Verification items for the finished model (mm, model axes). Coordinates: 2 decimals unless noted, no trailing zeros. Answer in a Markdown table with one row per item.
from build123d import *

# Parameters (mm, degrees)
F0_W     = 1375.41
F0_H     = 16.002
F0_R     = 2.286
F1_DEPTH = 3.175


with BuildPart() as f1:
    # F0 (on Top) → F1 (new body)
    with BuildSketch(Plane.XY):
        Rectangle(F0_W, F0_H)
        with Locations((-680.593, 0)):
            Circle(F0_R, mode=Mode.SUBTRACT)
        with Locations((-652.653, 0)):
            Circle(F0_R, mode=Mode.SUBTRACT)
        with Locations((-636.143, 0)):
            Circle(F0_R, mode=Mode.SUBTRACT)
        with Locations((-608.203, 0)):
            Circle(F0_R, mode=Mode.SUBTRACT)
        with Locations((-591.693, 0)):
            Circle(F0_R, mode=Mode.SUBTRACT)
        with Locations((-563.753, 0)):
            Circle(F0_R, mode=Mode.SUBTRACT)
        with Locations((-547.243, 0)):
            Circle(F0_R, mode=Mode.SUBTRACT)
        with Locations((-519.303, 0)):
            Circle(F0_R, mode=Mode.SUBTRACT)
        with Locations((-502.793, 0)):
            Circle(F0_R, mode=Mode.SUBTRACT)
        with Locations((-474.853, 0)):
            Circle(F0_R, mode=Mode.SUBTRACT)
        with Locations((-458.343, 0)):
            Circle(F0_R, mode=Mode.SUBTRACT)
        with Locations((-430.403, 0)):
            Circle(F0_R, mode=Mode.SUBTRACT)
        with Locations((-413.893, 0)):
            Circle(F0_R, mode=Mode.SUBTRACT)
        with Locations((-385.953, 0)):
            Circle(F0_R, mode=Mode.SUBTRACT)
        with Locations((-369.443, 0)):
            Circle(F0_R, mode=Mode.SUBTRACT)
        with Locations((-341.503, 0)):
            Circle(F0_R, mode=Mode.SUBTRACT)
        with Locations((-324.993, 0)):
            Circle(F0_R, mode=Mode.SUBTRACT)
        with Locations((-297.053, 0)):
            Circle(F0_R, mode=Mode.SUBTRACT)
        with Locations((-280.543, 0)):
            Circle(F0_R, mode=Mode.SUBTRACT)
        with Locations((-252.603, 0)):
            Circle(F0_R, mode=Mode.SUBTRACT)
        with Locations((-236.093, 0)):
            Circle(F0_R, mode=Mode.SUBTRACT)
        with Locations((-208.153, 0)):
            Circle(F0_R, mode=Mode.SUBTRACT)
        with Locations((-191.643, 0)):
            Circle(F0_R, mode=Mode.SUBTRACT)
        with Locations((-163.703, 0)):
            Circle(F0_R, mode=Mode.SUBTRACT)
        with Locations((-147.193, 0)):
            Circle(F0_R, mode=Mode.SUBTRACT)
        with Locations((-119.253, 0)):
            Circle(F0_R, mode=Mode.SUBTRACT)
        with Locations((-102.743, 0)):
            Circle(F0_R, mode=Mode.SUBTRACT)
        with Locations((-74.803, 0)):
            Circle(F0_R, mode=Mode.SUBTRACT)
        with Locations((-58.293, 0)):
            Circle(F0_R, mode=Mode.SUBTRACT)
        with Locations((-30.353, 0)):
            Circle(F0_R, mode=Mode.SUBTRACT)
        with Locations((-13.843, 0)):
            Circle(F0_R, mode=Mode.SUBTRACT)
        with Locations((14.097, 0)):
            Circle(F0_R, mode=Mode.SUBTRACT)
        with Locations((30.607, 0)):
            Circle(F0_R, mode=Mode.SUBTRACT)
        with Locations((58.547, 0)):
            Circle(F0_R, mode=Mode.SUBTRACT)
        with Locations((75.057, 0)):
            Circle(F0_R, mode=Mode.SUBTRACT)
        with Locations((102.997, 0)):
            Circle(F0_R, mode=Mode.SUBTRACT)
        with Locations((119.507, 0)):
            Circle(F0_R, mode=Mode.SUBTRACT)
        with Locations((147.447, 0)):
            Circle(F0_R, mode=Mode.SUBTRACT)
        with Locations((163.957, 0)):
            Circle(F0_R, mode=Mode.SUBTRACT)
        with Locations((191.897, 0)):
            Circle(F0_R, mode=Mode.SUBTRACT)
        with Locations((208.407, 0)):
            Circle(F0_R, mode=Mode.SUBTRACT)
        with Locations((236.347, 0)):
            Circle(F0_R, mode=Mode.SUBTRACT)
        with Locations((252.857, 0)):
            Circle(F0_R, mode=Mode.SUBTRACT)
        with Locations((280.797, 0)):
            Circle(F0_R, mode=Mode.SUBTRACT)
        with Locations((297.307, 0)):
            Circle(F0_R, mode=Mode.SUBTRACT)
        with Locations((325.247, 0)):
            Circle(F0_R, mode=Mode.SUBTRACT)
        with Locations((341.757, 0)):
            Circle(F0_R, mode=Mode.SUBTRACT)
        with Locations((369.697, 0)):
            Circle(F0_R, mode=Mode.SUBTRACT)
        with Locations((386.207, 0)):
            Circle(F0_R, mode=Mode.SUBTRACT)
        with Locations((414.147, 0)):
            Circle(F0_R, mode=Mode.SUBTRACT)
        with Locations((430.657, 0)):
            Circle(F0_R, mode=Mode.SUBTRACT)
        with Locations((458.597, 0)):
            Circle(F0_R, mode=Mode.SUBTRACT)
        with Locations((475.107, 0)):
            Circle(F0_R, mode=Mode.SUBTRACT)
        with Locations((503.047, 0)):
            Circle(F0_R, mode=Mode.SUBTRACT)
        with Locations((519.557, 0)):
            Circle(F0_R, mode=Mode.SUBTRACT)
        with Locations((547.497, 0)):
            Circle(F0_R, mode=Mode.SUBTRACT)
        with Locations((564.007, 0)):
            Circle(F0_R, mode=Mode.SUBTRACT)
        with Locations((591.947, 0)):
            Circle(F0_R, mode=Mode.SUBTRACT)
        with Locations((608.457, 0)):
            Circle(F0_R, mode=Mode.SUBTRACT)
        with Locations((636.397, 0)):
            Circle(F0_R, mode=Mode.SUBTRACT)
        with Locations((652.907, 0)):
            Circle(F0_R, mode=Mode.SUBTRACT)
        with Locations((680.847, 0)):
            Circle(F0_R, mode=Mode.SUBTRACT)
    extrude(amount=F1_DEPTH)


solid = f1.part
1) Thickness scan on L1, parallel to Y at x = -13.5, z = 0.2; L2, parallel to Y at x = 548, z = 1.85. Record the ranges inside material, lowest first. Write a range as [from, to].
Response values:
| item | result |
|---|---|
| L1 | y = [-8, -2.26], [2.26, 8] |
| L2 | y = [-8, -2.23], [2.23, 8] |
2) Sectioned sample at A-A (z = 2.45). Give the number of separate pieces and of enclosed holes in the cut face, then the cut area to 3 significant figures.
Response values:
| item | result |
|---|---|
| separate pieces | 1 |
| enclosed holes | 62 |
| area | 21,000 mm² |
3) Depth check by flat-ended pin: pin 1 (2.5 mm diameter, centred on x = 14.097, y = 0, fed in from +Z). Enter the tip coordinate at first touch or a pass-through.
Response values:
| item | result |
|---|---|
| pin 1 | passes through |
